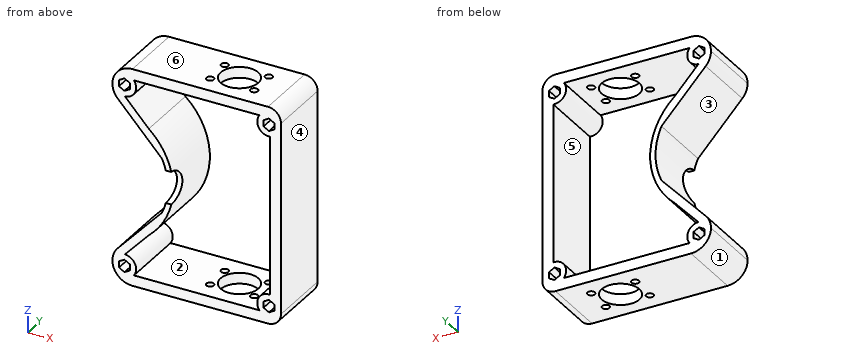
from build123d import *

# Parameters (mm, degrees)
SKETCH1_W               = 95.25
SKETCH1_H               = 6.35
BOSS_EXTRUDE1_DEPTH     = 38.1
SKETCH2_W               = 6.35
SKETCH2_H               = 127
BOSS_EXTRUDE2_DEPTH     = 38.1
SKETCH3_W               = 88.9
SKETCH3_H               = 6.35
BOSS_EXTRUDE3_DEPTH     = 38.1
SKETCH4_R               = 11
CUT_EXTRUDE1_DEPTH      = 149.412147835
SKETCH5_R               = 2.15265
CUT_EXTRUDE2_DEPTH      = 149.412147835
FILLET1_R               = 7.62
BOSS_EXTRUDE4_DEPTH     = 38.1
CUT_EXTRUDE8_REACH      = 171.022
CUT_EXTRUDE8_END_RADIUS = 38.1
FILLET2_R               = 11.688947
FILLET3_R               = 11.688947
FILLET4_R               = 6.35
SKETCH15_R              = 6.841174209
BOSS_EXTRUDE7_DEPTH     = 38.1
CUT_EXTRUDE12_DEPTH     = 157.640484095


with BuildPart() as part:
    # Sketch1 → Boss-Extrude1 (new body)
    with BuildSketch(Plane(origin=(0, 0, 0), x_dir=(1, 0, 0), z_dir=(0, 1, 0))):
        with Locations((19.05, 12.7)):
            Rectangle(SKETCH1_W, SKETCH1_H)
    extrude(amount=BOSS_EXTRUDE1_DEPTH)

    # Sketch2 → Boss-Extrude2 (add)
    with BuildSketch(Plane(origin=(0, 38.1, 0), x_dir=(1, 0, 0), z_dir=(0, 1, 0))):
        with Locations((63.5, 73.025)):
            Rectangle(SKETCH2_W, SKETCH2_H)
    extrude(amount=-BOSS_EXTRUDE2_DEPTH)

    # Sketch3 → Boss-Extrude3 (add)
    with BuildSketch(Plane(origin=(0, 38.1, 0), x_dir=(1, 0, 0), z_dir=(0, 1, 0))):
        with Locations((15.875, 133.35)):
            Rectangle(SKETCH3_W, SKETCH3_H)
    extrude(amount=-BOSS_EXTRUDE3_DEPTH)

    # Sketch4 → Cut-Extrude1 (cut, through all)
    with BuildSketch(Plane(origin=(0, 0, -136.525), x_dir=(-1, 0, 0), z_dir=(0, 0, -1))):
        with Locations((-31.75, 19.05)):
            Circle(SKETCH4_R)
    extrude(amount=-CUT_EXTRUDE1_DEPTH, mode=Mode.SUBTRACT)

    # Sketch5 → Cut-Extrude2 (cut, through all)
    with BuildSketch(Plane(origin=(0, 0, -136.525), x_dir=(-1, 0, 0), z_dir=(0, 0, -1))):
        with Locations((-18.877667779, 26.704865736)):
            Circle(SKETCH5_R)
        with Locations((-19.228536904, 10.833743663)):
            Circle(SKETCH5_R)
        with Locations((-44.622332221, 11.395134264)):
            Circle(SKETCH5_R)
        with Locations((-44.271463096, 27.266256337)):
            Circle(SKETCH5_R)
    extrude(amount=-CUT_EXTRUDE2_DEPTH, mode=Mode.SUBTRACT)

    # Fillet1
    fillet1_edges = [part.edges().sort_by_distance(p)[0] for p in [
        (66.675, 19.05, -136.525),
        (66.675, 19.05, -9.525),
    ]]
    fillet(fillet1_edges, radius=FILLET1_R)

    # Sketch10 → Boss-Extrude4 (add)
    with BuildSketch(Plane(origin=(0, 38.1, 0), x_dir=(1, 0, 0), z_dir=(0, 1, 0))):
        with BuildLine():
            Line((-28.575, 15.875), (-28.575, 9.525))
            Line((-28.575, 9.525), (-31.75, 9.525))
            Line((-31.75, 9.525), (-31.75, 25.781))
            Line((-31.75, 25.781), (-2.821027965, 57.15))
            ThreePointArc((-2.821027965, 57.15), (0.643811071, 73.025), (-2.821027965, 88.9))
            Line((-2.821027965, 88.9), (-31.75, 120.269))
            Line((-31.75, 120.269), (-31.75, 136.525))
            Line((-31.75, 136.525), (-28.575, 136.525))
            Line((-28.575, 136.525), (-28.575, 123.825))
            Line((-28.575, 123.825), (-10.494392478, 104.219375))
            ThreePointArc((-10.494392478, 104.219375), (3.775200806, 73.025), (-10.494392478, 41.830625))
            Line((-10.494392478, 41.830625), (-28.575, 22.225))
            Line((-28.575, 22.225), (-28.575, 15.875))
        make_face()
    extrude(amount=-BOSS_EXTRUDE4_DEPTH)

    # Cut-Extrude8: up to this cylinder (the profile starts outside it)
    cut_extrude8_end = Plane(origin=(-37.456188929, 4.042536, -73.025), z_dir=(0, 1, 0)) * Cylinder(CUT_EXTRUDE8_END_RADIUS, 419.244, mode=Mode.PRIVATE)
    # Sketch12 → Cut-Extrude8 (cut, up to the surface)
    with BuildSketch(Plane.ZY.offset(-60.325), mode=Mode.PRIVATE) as cut_extrude8_sk1:
        with BuildLine():
            Line((-82.55, 0), (-63.5, 0))
            ThreePointArc((-63.5, 0), (-73.025, 9.525), (-82.55, 0))
        make_face()
    cut_extrude8_tool1 = extrude(cut_extrude8_sk1.sketch, amount=CUT_EXTRUDE8_REACH, mode=Mode.PRIVATE) - cut_extrude8_end
    add(cut_extrude8_tool1.solids().sort_by_distance((60.325, 4.042536, -73.025))[0], mode=Mode.SUBTRACT)

    # Fillet2
    fillet2_edges = [part.edges().sort_by_distance(p)[0] for p in [
        (-31.75, 19.05, -136.525),
        (-31.75, 19.05, -120.269),
    ]]
    fillet(fillet2_edges, radius=FILLET2_R - 0.0001)  # a hair under: the kernel refuses the full size

    # Fillet3
    fillet3_edges = [part.edges().sort_by_distance(p)[0] for p in [
        (-31.75, 19.05, -25.781),
        (-31.75, 19.05, -9.525),
    ]]
    fillet(fillet3_edges, radius=FILLET3_R - 0.0001)  # a hair under: the kernel refuses the full size

    # Fillet4
    fillet4_edges = [part.edges().sort_by_distance(p)[0] for p in [
        (60.325, 19.05, -15.875),
        (60.325, 19.05, -130.175),
    ]]
    fillet(fillet4_edges, radius=FILLET4_R)

    # Sketch15 → Boss-Extrude7 (add)
    # profile 1 of 4: a face of its own
    with BuildSketch(Plane(origin=(0, 38.1, 0), x_dir=(1, 0, 0), z_dir=(0, 1, 0))):
        with Locations((59.652254611, 126.150383493)):
            Circle(SKETCH15_R)
        Polygon((59.652254611, 129.816557703), (56.477254611, 127.983470598), (56.477254611, 124.317296388), (59.652254611, 122.484209284), (62.827254611, 124.317296388), (62.827254611, 127.983470598), align=None, mode=Mode.SUBTRACT)
    # profile 2 of 4: a face of its own
    with BuildSketch(Plane(origin=(0, 38.1, 0), x_dir=(1, 0, 0), z_dir=(0, 1, 0))):
        with Locations((-24.727254611, 19.899616507)):
            Circle(SKETCH15_R)
        Polygon((-21.552254611, 21.732703612), (-24.727254611, 23.565790716), (-27.902254611, 21.732703612), (-27.902254611, 18.066529402), (-24.727254611, 16.233442297), (-21.552254611, 18.066529402), align=None, mode=Mode.SUBTRACT)
    # profile 3 of 4: a face of its own
    with BuildSketch(Plane(origin=(0, 38.1, 0), x_dir=(1, 0, 0), z_dir=(0, 1, 0))):
        with Locations((-24.727254611, 126.150383493)):
            Circle(SKETCH15_R)
        Polygon((-21.552254611, 127.983470598), (-21.552254611, 124.317296388), (-24.727254611, 122.484209284), (-27.902254611, 124.317296388), (-27.902254611, 127.983470598), (-24.727254611, 129.816557703), align=None, mode=Mode.SUBTRACT)
    # profile 4 of 4: a face of its own
    with BuildSketch(Plane(origin=(0, 38.1, 0), x_dir=(1, 0, 0), z_dir=(0, 1, 0))):
        with Locations((59.652254611, 19.899616507)):
            Circle(SKETCH15_R)
        Polygon((56.477254611, 18.066529402), (56.477254611, 21.732703612), (59.652254611, 23.565790716), (62.827254611, 21.732703612), (62.827254611, 18.066529402), (59.652254611, 16.233442297), align=None, mode=Mode.SUBTRACT)
    extrude(amount=-BOSS_EXTRUDE7_DEPTH)

    # Sketch21 → Cut-Extrude12 (cut, through all)
    with BuildSketch(Plane(origin=(0, 38.1, 0), x_dir=(1, 0, 0), z_dir=(0, 1, 0))):
        Polygon((-21.552254611, 21.732703612), (-24.727254611, 23.565790716), (-27.902254611, 21.732703612), (-27.902254611, 18.066529402), (-24.727254611, 16.233442297), (-21.552254611, 18.066529402), align=None)
        Polygon((56.477254611, 18.066529402), (56.477254611, 21.732703612), (59.652254611, 23.565790716), (62.827254611, 21.732703612), (62.827254611, 18.066529402), (59.652254611, 16.233442297), align=None)
        Polygon((59.652254611, 129.816557703), (56.477254611, 127.983470598), (56.477254611, 124.317296388), (59.652254611, 122.484209284), (62.827254611, 124.317296388), (62.827254611, 127.983470598), align=None)
        Polygon((-21.552254611, 127.983470598), (-21.552254611, 124.317296388), (-24.727254611, 122.484209284), (-27.902254611, 124.317296388), (-27.902254611, 127.983470598), (-24.727254611, 129.816557703), align=None)
    extrude(amount=-CUT_EXTRUDE12_DEPTH, mode=Mode.SUBTRACT)


solid = part.part
For this review, take the finished solid that the model builds, in its own axes (mm). Face numbers are marked on the shaded views. A direction names the side the tool comes from. Round coordinates to 2 decimals unless told otherwise and drop trailing zeros. Order: outer loops, then holes, each group sorted by start corner. A loop starts at its lowest first (then second) coordinate and runs counter-clockwise, first axis right, second up. Notation, with made-up numbers: M -30.75,-26.75 L -12.75,-26.75 A24 cw -12.75,-2.75 Z; hole C 25.25,71.25 d10. An arc over 180 degrees is marked long. Write each question's results on one line, items separated by ' | '. Start each with the question number.
1. To check wall thickness, follow L1, parallel to Z at x = 47.5, y = 3 (3 decimals); L2, parallel to X at y = 17.5, z = -74.5 (3 decimals); L3, parallel to Z at x = 60.5, y = 9. State the ranges of each line that lie inside material, in increasing order. Write a range as [from, to].
2. Add section A-A (x = 31.75). State the section outline as (y, z) points (3 decimals).
3. Tool access review of the marked faces 1, 2 and 3: name each direction out of +Z, -Z, +X, -X, +Y, -Y from which nothing blocks a thin tool from reaching the whole face with its end or side.
4. Add section C-C (y = 19.05). State how many separate pieces and enclosed holes the cut face has, then the cut area to 3 significant figures.
5. Add section B-B (z = -81). State the section outline as (x, y) points (3 decimals).
6. Add section D-D (x = 6). State the section outline as (y, z) points (3 decimals).
7. Clearance check with flat-ended pins moving along their axes: pin 1 Ø8 at (x, z) = (-20.5, -116) entering from +Y; pin 2 Ø1.8 at (y, z) = (21, -126.5) entering from -X (3 decimals). State where each tip first meets the part, or that it passes through.
8. Draft analysis for pull direction Z (two halves, no side actions). For the marked faces 4, 5 and 6, state which applies: pulls with the +Z half, pulls with the -Z half, needs draft (parallel to the pull), parting line crosses it, or undercut.
Output values:
1) L1: [-136.525, -130.175], [-15.875, -9.525] | L2: [0.615, 3.749], [60.325, 66.675] | L3: [-136.39, -129.33], [-122.97, -23.08], [-16.72, -9.66]
2) outline: M 0,-136.525 L 8.05,-136.525 L 8.05,-130.175 L 0,-130.175 Z; M 0,-15.875 L 8.05,-15.875 L 8.05,-9.525 L 0,-9.525 Z; M 30.05,-136.525 L 38.1,-136.525 L 38.1,-130.175 L 30.05,-130.175 Z; M 30.05,-15.875 L 38.1,-15.875 L 38.1,-9.525 L 30.05,-9.525 Z
3) face 1: -Z, -X, +Y, -Y | face 2: +Y, -Y | face 3: -X, +Y, -Y
4) separate pieces: 2 | enclosed holes: 4 | area: 2,360 mm^2
5) outline: M -0.2,5.208 L 2.997,5.208 L 2.997,38.1 L -0.2,38.1 Z; M 60.325,0 L 66.675,0 L 66.675,38.1 L 60.325,38.1 Z
6) outline: M 0,-136.525 L 38.1,-136.525 L 38.1,-130.175 L 0,-130.175 Z; M 0,-15.875 L 38.1,-15.875 L 38.1,-9.525 L 0,-9.525 Z
7) pin 1: y = 38.1 | pin 2: x = -31.725
8) face 4: needs draft | face 5: undercut | face 6: pulls with the +Z half
